from build123d import *

# Parameters (mm, degrees)
PAD003_DEPTH    = 18.5
SKETCH005_W     = 18
SKETCH005_H     = 190
POCKET_DEPTH    = 5.5
POCKET001_DEPTH = 8.5


with BuildPart() as part:
    # Clone2D002 → Pad003 (new body)
    with BuildSketch(Plane.XY):
        with BuildLine():
            Line((-151, 95), (-142, 95))
            Line((-142, 95), (-142, 68))
            Line((-142, 68), (-129, 68))
            Line((-129, 68), (-129, 95))
            Line((-129, 95), (129, 95))
            Line((129, 95), (129, 68))
            Line((129, 68), (142, 68))
            Line((142, 68), (142, 95))
            Line((142, 95), (151, 95))
            ThreePointArc((151, 95), (157.363961, 92.363961), (160, 86))
            Line((160, 86), (160, -86))
            ThreePointArc((160, -86), (157.363961, -92.363961), (151, -95))
            Line((151, -95), (142, -95))
            Line((142, -95), (142, -68))
            Line((142, -68), (129, -68))
            Line((129, -68), (129, -95))
            Line((129, -95), (-129, -95))
            Line((-129, -95), (-129, -68))
            Line((-129, -68), (-142, -68))
            Line((-142, -68), (-142, -95))
            Line((-142, -95), (-151, -95))
            ThreePointArc((-151, -95), (-157.363961, -92.363961), (-160, -86))
            Line((-160, -86), (-160, 86))
            ThreePointArc((-160, 86), (-157.363961, 92.363961), (-151, 95))
        make_face()
    extrude(amount=PAD003_DEPTH)

    # Sketch005 (on Face26 of Pad003) → Pocket (cut)
    with BuildSketch(Plane.XY.offset(18.5)):
        with Locations((-138, 0)):
            Rectangle(SKETCH005_W, SKETCH005_H)
    pocket = extrude(amount=-POCKET_DEPTH, mode=Mode.SUBTRACT)

    # Mirrored: Pocket across Sketch005 V_Axis
    add(pocket.mirror(Plane(origin=(0, 0, 18.5), x_dir=(0, 0, 1), z_dir=(1, 0, 0))), mode=Mode.SUBTRACT)

    # Sketch006 (on Face31 of Pocket) → Pocket001 (cut)
    with BuildSketch(Plane.XY.offset(18.5)):
        with BuildLine():
            Line((-112, 87), (112, 87))
            ThreePointArc((121, 78), (118.363961, 84.363961), (112, 87))
            Line((121, 78), (121, -78))
            ThreePointArc((112, -87), (118.363961, -84.363961), (121, -78))
            Line((112, -87), (-112, -87))
            ThreePointArc((-121, -78), (-118.363961, -84.363961), (-112, -87))
            Line((-121, -78), (-121, 78))
            ThreePointArc((-112, 87), (-118.363961, 84.363961), (-121, 78))
        make_face()
    pocket001 = extrude(amount=-POCKET001_DEPTH, mode=Mode.SUBTRACT)

    # Mirrored001: Pocket001 across Sketch006 V_Axis
    add(pocket001.mirror(Plane(origin=(0, 0, 18.5), x_dir=(0, 0, 1), z_dir=(1, 0, 0))), mode=Mode.SUBTRACT)


with BuildPart() as part_1:
    # Clone001 placement: moved
    add(part.part.moved(Location((0, 0, 35))))


solid = part_1.part
Input: part model. Units: mm. Frame: model coordinates. A direction names the side the tool comes from. Give positions to 0.01 mm unless a question says otherwise; leave off trailing zeros. Loops run counter-clockwise (first coordinate to the right, second up) from the corner with the lowest first, then second, coordinate; pieces in that order, holes last. Notation, with made-up numbers: (42, -11.75) -> (62, -11.75) arc R27 cw to (62, 26.25) -> close; hole circle Ø7 at (13.5, 9.5). An arc over 180 degrees is marked (long way). Answer as a JSON object with one key per item and string values. Group by question number.
Item 1: Cut plane D-D, the plane y = 0.5. Return the cut outline in (x, z).
Item 2: Pull-direction query (X, two-part tool) for faces 6 (the flat face through (147, -95, 42)), 7 (the cylindrical face through (118.434, 84.294, 49.31)), 8 (the cylindrical face through (157.434, -92.294, 44.12)), 9 (the flat face through (-2, 87, 49)); classes: released by +X, released by -X, zero draft, split by the parting line, or undercut.
Item 3: Reachability of faces 1 (the flat face through (-138, 1, 48)), 2 (the flat face through (146, 95, 42)), 3 (the flat face through (-135, -68, 41)), 4 (the flat face through (2, 1, 45)), 5 (the flat face through (135, 68, 41)) from +Z, -Z, +X, -X, +Y, -Y: full face, straight path, thin tool, end or side. Return the list, or none.
Item 4: Pin query (flat end, axial travel): P1, Ø5.5, axis at x = -135, y = -16.5, coming from the +Z side; P2, Ø5, axis at x = 98.5, y = 7, coming from the +Z side. Return the tip coordinate at first contact, or that it passes through.
Item 5: Cut plane C-C, the plane z = 38.5. Return the cut outline in (x, y).
Item 6: Cut plane A-A, the plane y = -83. Return the cut outline in (x, z), and give its area (3 significant figures).
Item 7: Cut plane B-B, the plane x = -109. Return the cut outline in (y, z), and give its area (3 significant figures).
Item 8: Line query: probe 1 along X at (y, z) = (-76.5, 40.5); probe 2 along X at (y, z) = (3, 49.25); probe 3 along X at (y, z) = (-4, 47.5). Output: solid intervals per line, ascending.
Checks:
{
 "1": {"outline": "(-160, 35) -> (160, 35) -> (160, 53.5) -> (147, 53.5) -> (147, 48) -> (129, 48) -> (129, 53.5) -> (121, 53.5) -> (121, 45) -> (-121, 45) -> (-121, 53.5) -> (-129, 53.5) -> (-129, 48) -> (-147, 48) -> (-147, 53.5) -> (-160, 53.5) -> close"},
 "2": {"face 6": "zero draft", "face 7": "undercut", "face 8": "released by +X", "face 9": "undercut"},
 "3": {"face 1": "+Z, +Y, -Y", "face 2": "+Z, -Z, +X, -X, +Y", "face 3": "+Z, -Z, -Y", "face 4": "+Z", "face 5": "+Z, -Z, +Y"},
 "4": {"P1": "stops at z = 48", "P2": "stops at z = 45"},
 "5": {"outline": "(-160, -86) arc R9 ccw to (-151, -95) -> (-142, -95) -> (-142, -68) -> (-129, -68) -> (-129, -95) -> (129, -95) -> (129, -68) -> (142, -68) -> (142, -95) -> (151, -95) arc R9 ccw to (160, -86) -> (160, 86) arc R9 ccw to (151, 95) -> (142, 95) -> (142, 68) -> (129, 68) -> (129, 95) -> (-129, 95) -> (-129, 68) -> (-142, 68) -> (-142, 95) -> (-151, 95) arc R9 ccw to (-160, 86) -> close"},
 "6": {"outline": "(-160, 35) -> (-142, 35) -> (-142, 48) -> (-147, 48) -> (-147, 53.5) -> (-160, 53.5) -> close; (-129, 35) -> (129, 35) -> (129, 53.5) -> (119.48, 53.5) -> (119.48, 45) -> (-119.48, 45) -> (-119.48, 53.5) -> (-129, 53.5) -> close; (142, 35) -> (160, 35) -> (160, 53.5) -> (147, 53.5) -> (147, 48) -> (142, 48) -> close", "area": "3,350 mm²"},
 "7": {"outline": "(-95, 35) -> (95, 35) -> (95, 53.5) -> (87, 53.5) -> (87, 45) -> (-87, 45) -> (-87, 53.5) -> (-95, 53.5) -> close", "area": "2,040 mm²"},
 "8": {"probe 1": "x = -160 to -142, -129 to 129, 142 to 160", "probe 2": "x = -160 to -147, -129 to -121, 121 to 129, 147 to 160", "probe 3": "x = -160 to -121, 121 to 160"}
}
